Geometry: final body of the model. Coordinates: model frame, mm. Round coordinates to 2 decimals unless told otherwise and drop trailing zeros. Loops run counter-clockwise (first coordinate to the right, second up) from the corner with the lowest first, then second, coordinate; pieces in that order, holes last. Notation, with made-up numbers: (17, 66) - (30, 66) arc R15 ccw to (30, 79) - close; hole circle Ø3 at (45.25, -12.75). An arc over 180 degrees is marked (long way). Answer in a Markdown table with one row per item. Add a question column.
from build123d import *

# Parameters (mm, degrees)
F0_W     = 38.1
F0_H     = 88.9
F1_DEPTH = 914.4
F3_DEPTH = 88.9
F4_R     = 5.08


with BuildPart() as f1:
    # F0 (on Front) → F1 (new body)
    with BuildSketch(Plane.XZ):
        with Locations((-4.357182, 2.600797)):
            Rectangle(F0_W, F0_H)
    extrude(amount=F1_DEPTH)

    # F2 (on face) → F3 (cut)
    with BuildSketch(Plane.XY.offset(47.050797)):
        Polygon((-23.407182, -914.4), (14.692818, -914.4), (-23.407182, -876.3), align=None)
        Polygon((-23.407182, -38.1), (14.692818, 0), (-23.407182, 0), align=None)
    extrude(amount=-F3_DEPTH, mode=Mode.SUBTRACT)

    # F4
    f4_edges = [f1.edges().sort_by_distance(p)[0] for p in [
        (-23.407182, -457.2, 47.050797),
        (14.692818, -457.2, 47.050797),
        (-23.407182, -457.2, -41.849203),
        (14.692818, -457.2, -41.849203),
    ]]
    fillet(f4_edges, radius=F4_R)


solid = f1.part
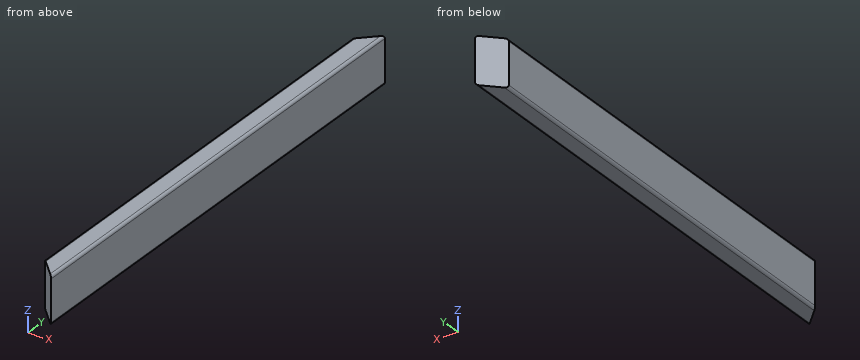
1) Material intervals for line 1 along X through (y, z) = (-167.5, -37); line 2 along Y through (x, z) = (-7, 9); line 3 along Y through (x, z) = (-7.5, 23.5), sorted ascending. Write a range as from..to.
2) Section A-A, the plane z = -6. Return the cut outline in (x, y), and give its area (3 significant figures).
3) Contact query for flat-ended pins moving along their axis: pin 1 Ø8 at (x, z) = (-9.5, -10) entering from +Y; pin 2 Ø8 at (x, z) = (9, -26) entering from +Y; pin 3 Ø1 at (x, z) = (-9, 11.5) entering from -Y. Output: stop coordinate, or through.
4) Section B-B, the plane x = -6. Return the cut outline in (y, z), and give its area (3 significant figures).
Evaluation:
| question | item | result |
|---|---|---|
| 1 | line 1 | x = -23.4..14.69 |
| 1 | line 2 | y = -892.71..-21.69 |
| 1 | line 3 | y = -892.21..-22.19 |
| 2 | outline | (-23.41, -876.3) - (14.69, -914.4) - (14.69, 0) - (-23.41, -38.1) - close |
| 2 | area | 33,400 mm² |
| 3 | pin 1 | stops at y = -20.19 |
| 3 | pin 2 | stops at y = -1.69 |
| 3 | pin 3 | stops at y = -891.21 |
| 4 | outline | (-893.71, -41.85) - (-20.69, -41.85) - (-20.69, 47.05) - (-893.71, 47.05) - close |
| 4 | area | 77,600 mm² |
